```python
from build123d import *

# Parameters (mm, degrees)
SKETCH1_W           = 42
SKETCH1_H           = 51
BOSS_EXTRUDE1_DEPTH = 5
SKETCH3_W           = 42
SKETCH3_H           = 51
SKETCH3_W_2         = 35
SKETCH3_H_2         = 45.75
BOSS_EXTRUDE3_DEPTH = 25
SKETCH4_R           = 8.75
CUT_EXTRUDE2_DEPTH  = 5
CUT_EXTRUDE3_DEPTH  = 4
SKETCH7_W           = 6
SKETCH7_H           = 25
CUT_EXTRUDE4_DEPTH  = 4
SKETCH9_R           = 11
CUT_EXTRUDE5_DEPTH  = 4
SKETCH16_W          = 7
SKETCH16_H          = 30
BOSS_EXTRUDE5_DEPTH = 1.5
SKETCH17_W          = 7
SKETCH17_H          = 30
BOSS_EXTRUDE6_DEPTH = 1.5
SKETCH19_W          = 7
SKETCH19_H          = 30
BOSS_EXTRUDE7_DEPTH = 1.5
SKETCH18_R          = 1.4
CUT_EXTRUDE7_DEPTH  = 6
BOSS_EXTRUDE8_DEPTH = 30
SKETCH24_W          = 30
SKETCH24_H          = 20
CUT_EXTRUDE8_DEPTH  = 32
SKETCH29_R          = 1.4
CUT_EXTRUDE9_DEPTH  = 6
CUT_EXTRUDE10_DEPTH = 6
SKETCH28_R          = 2.5
SKETCH28_R_2        = 1.4
CUT_EXTRUDE11_DEPTH = 6


with BuildPart() as part:
    # Sketch1 → Boss-Extrude1 (new body)
    with BuildSketch(Plane(origin=(0, 0, 0), x_dir=(1, 0, 0), z_dir=(0, 1, 0))):
        Rectangle(SKETCH1_W, SKETCH1_H)
    extrude(amount=BOSS_EXTRUDE1_DEPTH)

    # Sketch3 → Boss-Extrude3 (add)
    with BuildSketch(Plane(origin=(0, 5, 0), x_dir=(1, 0, 0), z_dir=(0, 1, 0))):
        Rectangle(SKETCH3_W, SKETCH3_H)
        Rectangle(SKETCH3_W_2, SKETCH3_H_2, mode=Mode.SUBTRACT)
    extrude(amount=BOSS_EXTRUDE3_DEPTH)

    # Sketch4 → Cut-Extrude2 (cut)
    with BuildSketch(Plane.ZY.offset(21)):
        with Locations((-12.5, 17.5)):
            Circle(SKETCH4_R)
    extrude(amount=-CUT_EXTRUDE2_DEPTH, mode=Mode.SUBTRACT)

    # Sketch6 → Cut-Extrude3 (cut)
    with BuildSketch(Plane(origin=(-17.5, 0, 0), x_dir=(0, 0, -1), z_dir=(1, 0, 0))):
        with BuildLine():
            Line((9.375, 17.5), (9.375, 30))
            Line((9.375, 30), (15.625, 30))
            Line((15.625, 30), (15.625, 17.5))
            ThreePointArc((15.625, 17.5), (12.5, 14.375), (9.375, 17.5))
        make_face()
    extrude(amount=-CUT_EXTRUDE3_DEPTH, mode=Mode.SUBTRACT)

    # Sketch7 → Cut-Extrude4 (cut)
    with BuildSketch(Plane.ZY.offset(21)):
        with Locations((2, 17.5)):
            Rectangle(SKETCH7_W, SKETCH7_H)
    extrude(amount=-CUT_EXTRUDE4_DEPTH, mode=Mode.SUBTRACT)

    # Sketch9 → Cut-Extrude5 (cut)
    with BuildSketch(Plane(origin=(21, 0, 0), x_dir=(0, 0, -1), z_dir=(1, 0, 0))):
        with Locations((12.5, 17.5)):
            Circle(SKETCH9_R)
    extrude(amount=-CUT_EXTRUDE5_DEPTH, mode=Mode.SUBTRACT)

    # Sketch16 → Boss-Extrude5 (add)
    with BuildSketch(Plane.ZY.offset(21)):
        with Locations((12, 15)):
            Rectangle(SKETCH16_W, SKETCH16_H)
    extrude(amount=BOSS_EXTRUDE5_DEPTH)

    # Sketch17 → Boss-Extrude6 (add)
    with BuildSketch(Plane(origin=(21, 0, 0), x_dir=(0, 0, -1), z_dir=(1, 0, 0))):
        with Locations((-12, 15)):
            Rectangle(SKETCH17_W, SKETCH17_H)
    extrude(amount=BOSS_EXTRUDE6_DEPTH)

    # Sketch19 → Boss-Extrude7 (add)
    with BuildSketch(Plane(origin=(0, 0, -25.5), x_dir=(-1, 0, 0), z_dir=(0, 0, -1))):
        with Locations((0, 15)):
            Rectangle(SKETCH19_W, SKETCH19_H)
    extrude(amount=BOSS_EXTRUDE7_DEPTH)

    # Sketch18 → Cut-Extrude7 (cut)
    with BuildSketch(Plane(origin=(0, 30, 0), x_dir=(1, 0, 0), z_dir=(0, 1, 0))):
        with Locations(Location((-20, -12, 0), (0, 0, 270))):
            Circle(SKETCH18_R)
        with Locations(Location((20, -12, 0), (0, 0, 90))):
            Circle(SKETCH18_R)
        with Locations(Location((0, 24.9375, 0), (0, 0, 270))):
            Circle(SKETCH18_R)
    extrude(amount=-CUT_EXTRUDE7_DEPTH, mode=Mode.SUBTRACT)

    # Sketch1_3 → Boss-Extrude8 (add)
    with BuildSketch(Plane(origin=(0, 0, 0), x_dir=(1, 0, 0), z_dir=(0, 1, 0))):
        Polygon((-11, -25.5), (-16, -25.5), (-16, -40.5), (-23, -40.5), (-23, -45.5), (-16, -45.5), (-16, -55.5), (-23, -55.5), (-23, -60.5), (24, -60.5), (24, -100.5), (29, -100.5), (29, -55.5), (16, -55.5), (16, -25.5), (11, -25.5), (11, -55.5), (-11, -55.5), align=None)
    extrude(amount=BOSS_EXTRUDE8_DEPTH)

    # Sketch24 → Cut-Extrude8 (cut)
    with BuildSketch(Plane.ZY.offset(16)):
        with Locations((40.5, 15)):
            Rectangle(SKETCH24_W, SKETCH24_H)
    extrude(amount=-CUT_EXTRUDE8_DEPTH, mode=Mode.SUBTRACT)

    # Sketch29 → Cut-Extrude9 (cut)
    with BuildSketch(Plane.ZY.offset(23)):
        with Locations((58, 25)):
            Circle(SKETCH29_R)
        with Locations(Location((43, 25, 0), (0, 0, 180))):
            Circle(SKETCH29_R)
        with Locations(Location((58, 5, 0), (0, 0, 180))):
            Circle(SKETCH29_R)
        with Locations((43, 5)):
            Circle(SKETCH29_R)
    extrude(amount=-CUT_EXTRUDE9_DEPTH, mode=Mode.SUBTRACT)

    # Sketch30 → Cut-Extrude10 (cut)
    with BuildSketch(Plane(origin=(29, 0, 0), x_dir=(0, 0, -1), z_dir=(1, 0, 0))):
        with BuildLine():
            ThreePointArc((-100.5, 15), (-96.106601718, 25.606601718), (-85.5, 30))
            Line((-85.5, 30), (-100.5, 30))
            Line((-100.5, 30), (-100.5, 15))
        make_face()
        with BuildLine():
            ThreePointArc((-85.5, 0), (-96.106601718, 4.393398282), (-100.5, 15))
            Line((-100.5, 15), (-100.5, 0))
            Line((-100.5, 0), (-85.5, 0))
        make_face()
    extrude(amount=-CUT_EXTRUDE10_DEPTH, mode=Mode.SUBTRACT)

    # Sketch28 → Cut-Extrude11 (cut)
    with BuildSketch(Plane.ZY.offset(-24)):
        with Locations((90.5, 15)):
            Circle(SKETCH28_R)
        with Locations((90.5, 22)):
            Circle(SKETCH28_R_2)
        with Locations((83.5, 15)):
            Circle(SKETCH28_R_2)
        with Locations(Location((90.5, 8, 0), (0, 0, 180))):
            Circle(SKETCH28_R_2)
        with Locations(Location((97.5, 15, 0), (0, 0, 180))):
            Circle(SKETCH28_R_2)
    extrude(amount=-CUT_EXTRUDE11_DEPTH, mode=Mode.SUBTRACT)


solid = part.part
```
Can you work these out from the model? Positions are in its coordinate system, mm. A direction names the side the tool comes from. Give positions to 0.01 mm unless a question says otherwise; leave off trailing zeros. Write each loop counter-clockwise with the first axis right and the second up, starting at its lowest first coordinate (ties: lowest second). Pieces come first, ordered by that corner, then holes. Notation, with made-up numbers: (-29.5, -0.75) - (-15.5, -0.75) arc R19 cw to (-15.5, 20.25) - close; hole circle Ø10 at (38, 39). An arc over 180 degrees is marked (long way). Write item = value, one per line. Start each with the question number.
1. Please list where these lines run through material, in increasing order: line 1 (Y direction, x = -19.1, z = 58); line 2 (Z direction, x = 18.15, y = 17.5); line 3 (Z direction, x = 16.5, y = 28) (3 decimals).
2. Imagine slicing it at A-A (z = 29.5). Please give me the cut outline in (x, y), and give its area (3 significant figures).
3. For pin 1 (3.5 mm diameter, centred on y = 9.5, z = 13.5, fed in from -X); pin 2 (9 mm diameter, centred on y = 21, z = 88, fed in from -X); pin 3 (5 mm diameter, centred on y = 9.5, z = 20, fed in from -X); pin 4 (3 mm diameter, centred on x = -19.5, z = 12.5, fed in from +Y), each with a flat end and sliding along its axis, tell me the tip position at first contact or that it passes through.
4. On a 3-axis mill with a long thin cutter (end or side, diameter ignored), from which of +Z, -Z, +X, -X, +Y, -Y can I reach the whole of each face in a straight line? I mean faces 1 (the face through (-12, 15, -25.5)), 2 (the face through (24, 15, 80)), 3 (the face through (19.028, 20.804, -22.992)). Say none if no direction works.
5. Thinking about a two-plate mould opening in X: for faces 4 (the face through (-21, 8, -8)), 5 (the face through (0, 17, -22.875)), 6 (the face through (26.46, 21.15, 89.39)), 7 (the face through (-11, 2, 41)), which applies, released by +X, released by -X, zero draft, split by the parting line, or undercut?
6. Imagine slicing it at D-D (z = 12). Please give me the cut outline in (x, y), and give its area (3 significant figures).
7. Imagine slicing it at B-B (x = 8). Please give me the cut outline in (y, z) (3 decimals).
8. Imagine slicing it at C-C (z = 97.5). Please give me the cut outline in (x, y).
Worked answers:
q1.line_1 = 0 to 3.6, 6.4 to 23.6, 26.4 to 30
q1.line_2 = -25.5 to -23.5, -1.5 to 25.5, 55.5 to 60.5
q1.line_3 = -25.5 to -22.875, 22.875 to 25.5, 55.5 to 60.5
q2.outline = (-16, 0) - (-11, 0) - (-11, 5) - (-16, 5) - close; (-16, 25) - (-11, 25) - (-11, 30) - (-16, 30) - close; (11, 0) - (16, 0) - (16, 5) - (11, 5) - close; (11, 25) - (16, 25) - (16, 30) - (11, 30) - close
q2.area = 100 mm2
q3.pin_1 = -22.5
q3.pin_2 = 24
q3.pin_3 = -21
q3.pin_4 = 30
q4.face_1 = -Z, -X, +Y, -Y
q4.face_2 = +Z, -X, +Y, -Y
q4.face_3 = +X
q5.face_4 = released by -X
q5.face_5 = undercut
q5.face_6 = zero draft
q5.face_7 = undercut
q6.outline = (-22.5, 0) - (22.5, 0) - (22.5, 30) - (21.4, 30) - (21.4, 24) - (18.6, 24) - (18.6, 30) - (17.5, 30) - (17.5, 5) - (-17.5, 5) - (-17.5, 30) - (-18.6, 30) - (-18.6, 24) - (-21.4, 24) - (-21.4, 30) - (-22.5, 30) - close
q6.area = 441 mm2
q7.outline = (0, -25.5) - (30, -25.5) - (30, -22.875) - (5, -22.875) - (5, 22.875) - (30, 22.875) - (30, 25.5) - (0, 25.5) - close; (0, 55.5) - (30, 55.5) - (30, 60.5) - (0, 60.5) - close
q8.outline = (24, 6) - (29, 6) - (29, 13.6) - (24, 13.6) - close; (24, 16.4) - (29, 16.4) - (29, 24) - (24, 24) - close
